Could you check a few things on this model? Use its own coordinates, in mm. Face numbers are marked on the shaded views. A direction names the side the tool comes from. Give positions to 0.01 mm unless a question says otherwise; leave off trailing zeros. Loops run counter-clockwise (first coordinate to the right, second up) from the corner with the lowest first, then second, coordinate; pieces in that order, holes last. Notation, with made-up numbers: (56, -23.5) -> (101, -23.5) arc R33 cw to (101, 8.5) -> close; hole circle Ø7 at (56, 66). An arc over 180 degrees is marked (long way). Put each result on its own line as item: value.
```python
from build123d import *

# Parameters (mm, degrees)
F1_DEPTH = 96
F2_W     = 43.5
F2_H     = 5
F3_DEPTH = 46
F4_W     = 47
F4_H     = 5
F5_DEPTH = 46
F6_W     = 43.5
F6_H     = 5
F7_DEPTH = 46
F9_D     = 14
F11_D    = 14
F13_D    = 14


with BuildPart() as f1:
    # F0 (on Top) → F1 (new body)
    with BuildSketch(Plane.XY):
        Polygon((-21, -21.505648), (-21, 19.494352), (-23.5, 19.494352), (-23.5, -24.005648), (23.5, -24.005648), (23.5, 19.494352), (21, 19.494352), (21, -21.505648), align=None)
    extrude(amount=F1_DEPTH)

    # F2 (on face) → F3 (join)
    with BuildSketch(Plane.YZ.offset(23.5)):
        with Locations((-2.255648, 2.5)):
            Rectangle(F2_W, F2_H)
    extrude(amount=F3_DEPTH)

    # F4 (on face) → F5 (join)
    with BuildSketch(Plane.XZ.offset(24.005648)):
        with Locations((0, 2.5)):
            Rectangle(F4_W, F4_H)
    extrude(amount=F5_DEPTH)

    # F6 (on face) → F7 (join)
    with BuildSketch(Plane(origin=(-23.5, 0, 0), x_dir=(0, -1, 0), z_dir=(-1, 0, 0))):
        with Locations((2.255648, 2.5)):
            Rectangle(F6_W, F6_H)
    extrude(amount=F7_DEPTH)

    # F9 (through all)
    with Locations(Plane.XY.offset(5)):
        with Locations((-48.5, -2.255648), (0, -49.005648), (48.5, -2.255648)):
            Hole(F9_D / 2)

    # F11 (through all)
    with Locations(Plane.XZ.offset(24.005648)):
        with Locations((0, 75), (0, 27)):
            Hole(F11_D / 2)

    # F13 (through all)
    with Locations(Plane.YZ.offset(23.5)):
        with Locations((-2.255648, 75), (-2.255648, 27)):
            Hole(F13_D / 2)


solid = f1.part
```
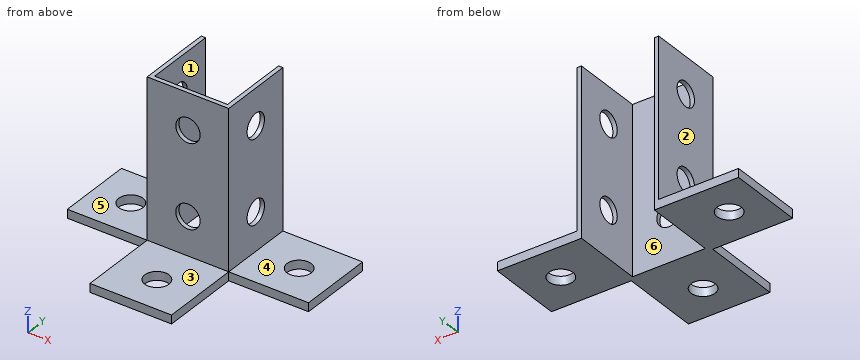
1. I need wall thicknesses on line 1 (X direction, y = 3, z = 83); line 2 (Z direction, x = -33, y = 14); line 3 (Y direction, x = -18.5, z = 64). Which ranges of each line are inside material? Lowest first, please.
Recorded:
line 1: x = -23.5 to -21, 21 to 23.5
line 2: z = 0 to 5
line 3: y = -24.01 to -21.51
2. If we section it at D-D (y = -44.5): List the corners of the cut face in (x, z) for me.
Recorded:
outline: (-23.5, 0) -> (-5.36, 0) -> (-5.36, 5) -> (-23.5, 5) -> close; (5.36, 0) -> (23.5, 0) -> (23.5, 5) -> (5.36, 5) -> close
3. For the marked faces 4, 5 and 6, which set-ups out of +Z, -Z, +X, -X, +Y, -Y let a thin tool reach every point of the face, with its end or its side?
Recorded:
face 4: +Z, +X, +Y, -Y
face 5: +Z, -X, +Y, -Y
face 6: +Z, -Z, +Y
4. I'm going to push flat-ended pins straight in: pin 1 (6 mm diameter, centred on x = 4.5, z = 82.5, fed in from +Y); pin 2 (3 mm diameter, centred on y = -22, z = 78.5, fed in from +X); pin 3 (2.5 mm diameter, centred on y = -36, z = 3, fed in from -X). Where does each tip first touch, or does it pass through?
Recorded:
pin 1: stops at y = -21.51
pin 2: stops at x = 23.5
pin 3: stops at x = -23.5
5. If we section it at B-B (z = 75): List the corners of the cut face in (x, y) for me, then the cut area to 4 significant figures.
Recorded:
outline: (-23.5, -24.01) -> (-7, -24.01) -> (-7, -21.51) -> (-21, -21.51) -> (-21, -9.26) -> (-23.5, -9.26) -> close; (-23.5, 4.74) -> (-21, 4.74) -> (-21, 19.49) -> (-23.5, 19.49) -> close; (7, -24.01) -> (23.5, -24.01) -> (23.5, -9.26) -> (21, -9.26) -> (21, -21.51) -> (7, -21.51) -> close; (21, 4.74) -> (23.5, 4.74) -> (23.5, 19.49) -> (21, 19.49) -> close
area: 217.5 mm^2
6. If we section it at C-C (x = 0): List the corners of the cut face in (y, z) for me.
Recorded:
outline: (-70.01, 0) -> (-56.01, 0) -> (-56.01, 5) -> (-70.01, 5) -> close; (-42.01, 0) -> (-21.51, 0) -> (-21.51, 20) -> (-24.01, 20) -> (-24.01, 5) -> (-42.01, 5) -> close; (-24.01, 34) -> (-21.51, 34) -> (-21.51, 68) -> (-24.01, 68) -> close; (-24.01, 82) -> (-21.51, 82) -> (-21.51, 96) -> (-24.01, 96) -> close
7. If we section it at A-A (x = 48.5): List the corners of the cut face in (y, z) for me, then the cut area to 4 significant figures.
Recorded:
outline: (-24.01, 0) -> (-9.26, 0) -> (-9.26, 5) -> (-24.01, 5) -> close; (4.74, 0) -> (19.49, 0) -> (19.49, 5) -> (4.74, 5) -> close
area: 147.5 mm^2
8. Thinking about a two-plate mould opening in X: for the marked faces 1, 2 and 3, which applies, pulls with the +X half, pulls with the -X half, needs draft (parallel to the pull), parting line crosses it, or undercut?
Recorded:
face 1: undercut
face 2: pulls with the -X half
face 3: needs draft
